from build123d import *

# Parameters (mm, degrees)
F1_DEPTH = 150
F3_R     = 3
F4_DEPTH = 25


with BuildPart() as f1:
    # F0 (on Front) → F1 (new body)
    with BuildSketch(Plane.XZ):
        with BuildLine():
            Line((0, -6), (0, 0))
            Line((0, 0), (-26.600782156, 0))
            ThreePointArc((-26.600782156, 0), (-27.0968220332, -1.3183717037), (-28.338886105, -1.9827784693))
            Line((-28.338886105, -1.9827784693), (-55.0189449519, -1.9827784693))
            Line((-55.0189449519, -1.9827784693), (-51.0017234212, -6))
            Line((-51.0017234212, -6), (0, -6))
        make_face()
    extrude(amount=F1_DEPTH)

    # F3 (on offset) → F4 (cut)
    with BuildSketch(Plane.XY):
        with Locations((-15, -15)):
            Circle(F3_R)
        with Locations((-15, -135)):
            Circle(F3_R)
        with Locations((-15, -75)):
            Circle(F3_R)
    extrude(amount=-F4_DEPTH, mode=Mode.SUBTRACT)


solid = f1.part
Could you check a few things on this model? Use its own coordinates, in mm. A direction names the side the tool comes from. Give positions to 0.01 mm unless a question says otherwise; leave off trailing zeros. Loops run counter-clockwise (first coordinate to the right, second up) from the corner with the lowest first, then second, coordinate; pieces in that order, holes last. Notation, with made-up numbers: M 31,15.5 L 50,15.5 A24 ccw 50,46.5 Z; hole C -38.5,89.25 d2. An arc over 180 degrees is marked long. Answer as a JSON object with one key per item and string values.
Q1. Suppose I cut it at A-A, the plane x = -15. List the corners of the cut face in (y, z) for me.
Values found:
{"outline": "M -150,-6 L -138,-6 L -138,0 L -150,0 Z; M -132,-6 L -78,-6 L -78,0 L -132,0 Z; M -72,-6 L -18,-6 L -18,0 L -72,0 Z; M -12,-6 L 0,-6 L 0,0 L -12,0 Z"}
Q2. If we mould it in two halves opening along X, with no side actions, what happens to faces 1 (the flat face through (-10, -74, 0)), 2 (the cylindrical face through (-15.65, -77.93, -2.96)), 3 (the flat face through (0, -74, -3))? For each: pulls with the +X half, pulls with the -X half, needs draft (parallel to the pull), parting line crosses it, or undercut.
Values found:
{"face 1": "needs draft", "face 2": "undercut", "face 3": "pulls with the +X half"}
Q3. For faces 4 (the flat face through (-41, -74, -1.983)), 5 (the flat face through (-26, -74, -6)), which set-ups out of +Z, -Z, +X, -X, +Y, -Y let a thin tool reach every point of the face, with its end or its side?
Values found:
{"face 4": "+Z, -X, +Y, -Y", "face 5": "-Z, +X, -X, +Y, -Y"}
Q4. Suppose I cut it at D-D, the plane x = -34. List the corners of the cut face in (y, z) for me.
Values found:
{"outline": "M -150,-6 L 0,-6 L 0,-1.98 L -150,-1.98 Z"}
Q5. For P1, Ø8, axis at x = -43, y = -25, coming from the +Z side; P2, Ø5, axis at x = -15, y = -135, coming from the -Z side; P3, Ø1.5, axis at y = -108, z = -3, coming from the -X side, each with a flat end and sliding along its axis, tell me the tip position at first contact or that it passes through.
Values found:
{"P1": "stops at z = -1.98", "P2": "passes through", "P3": "stops at x = -54.75"}
Q6. Suppose I cut it at C-C, the plane z = -4.25. List the corners of the cut face in (x, y) for me.
Values found:
{"outline": "M -52.75,-150 L 0,-150 L 0,0 L -52.75,0 Z; hole C -15,-135 d6; hole C -15,-75 d6; hole C -15,-15 d6"}
Q7. Suppose I cut it at B-B, the plane y = -15. List the corners of the cut face in (x, z) for me, plus the area to 3 significant figures.
Values found:
{"outline": "M -55.02,-1.98 L -51,-6 L -18,-6 L -18,0 L -26.6,0 A2 cw -28.34,-1.98 Z; M -12,-6 L 0,-6 L 0,0 L -12,0 Z", "area": "231 mm²"}
Q8. If I drill on probe 1 along Y at (x, z) = (-15, -4.05); probe 2 along Z at (x, y) = (-41, -62); probe 3 along X at (y, z) = (-135, -4.2), over which ranges is the centre line in solid material (lowest first)? Write a range as [from, to].
Values found:
{"probe 1": "y = [-150, -138], [-132, -78], [-72, -18], [-12, 0]", "probe 2": "z = [-6, -1.98]", "probe 3": "x = [-52.8, -18], [-12, 0]"}
